from build123d import *

# Parameters (mm, degrees)
F0_W          = 40
F0_H          = 70
F1_DEPTH      = 20
F1_DEPTH_BACK = 20
F3_D          = 19.5
F5_D          = 30
F6_R          = 19.99999


# Not quite as in the source:
# - a fillet or chamfer is up to 0.001 mm smaller than in the source, because OpenCascade refuses the exact size


with BuildPart() as f1:
    # F0 (on Front) → F1 (new body, two sides)
    with BuildSketch(Plane.XZ) as f1_sk:
        Rectangle(F0_W, F0_H)
    extrude(amount=F1_DEPTH)
    extrude(f1_sk.sketch, amount=-F1_DEPTH_BACK)

    # F3 (through all)
    with Locations(Plane(origin=(-20, 0, 0), x_dir=(0, -1, 0), z_dir=(-1, 0, 0))):
        with Locations((0, 20)):
            Hole(F3_D / 2)

    # F5 (through all)
    with Locations(Plane.XZ.offset(20)):
        with Locations((0, -15)):
            Hole(F5_D / 2)

    # F6 (radius 20 in the source; OpenCascade refuses exactly that, so slightly less here)
    f6_edges = [f1.edges().sort_by_distance(p)[0] for p in [
        (20, 0, -35),
        (-20, 0, -35),
    ]]
    fillet(f6_edges, radius=F6_R)


solid = f1.part
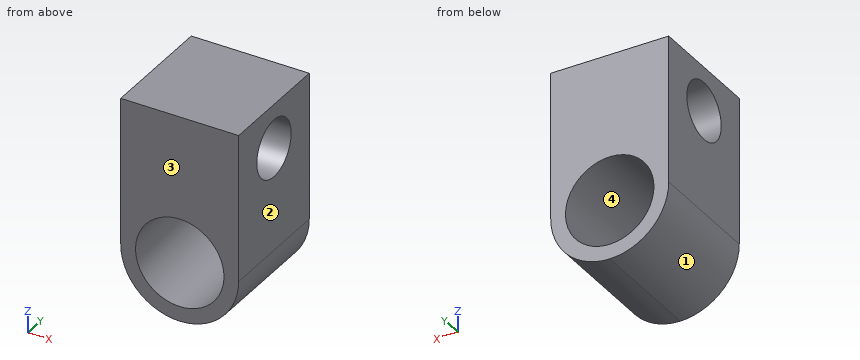
Design review of the part built by this model. Coordinates are the model's own, in mm. Face numbers are marked on the shaded views. Coordinates: 2 decimals unless noted, no trailing zeros. Order: outer loops, then holes, each group sorted by start corner. A loop starts at its lowest first (then second) coordinate and runs counter-clockwise, first axis right, second up. Notation, with made-up numbers: (-38.5, -16) - (8.5, -16) arc R32 ccw to (8.5, 10) - close; hole circle Ø8 at (-20, 2.25). An arc over 180 degrees is marked (long way). Put each result on its own line as item: value.
1) Take a section at C-C, the plane y = 0. Count the separate pieces of the cut face and the enclosed holes in it, and give its area (3 significant figures).
Response values:
separate pieces: 2
enclosed holes: 1
area: 1,140 mm²
2) The part is to be moulded in two halves that separate along X. For the marked faces 1, 2, 3 and 4, say which applies: released by +X, released by -X, zero draft, split by the parting line, or undercut.
Response values:
face 1: released by -X
face 2: released by +X
face 3: zero draft
face 4: undercut
3) Insertion check: P1, Ø1, axis at y = 10.5, z = -27, coming from the +X side; P2, Ø3, axis at y = 13, z = -21, coming from the -X side; P3, Ø18, axis at x = 0, z = -15, coming from the -Y side. Each pin has a flat end and moves straight along its axis. Give the tip position at first contact, or say it passes through.
Response values:
P1: stops at x = 16.36
P2: stops at x = -19.49
P3: passes through
4) Take a section at A-A, the plane z = 20. Give the boundary of the cut face in (x, y).
Response values:
outline: (-20, -20) - (20, -20) - (20, -9.75) - (-20, -9.75) - close; (-20, 9.75) - (20, 9.75) - (20, 20) - (-20, 20) - close
5) Take a section at B-B, the plane x = -1. Give the boundary of the cut face in (y, z).
Response values:
outline: (-20, -34.97) - (20, -34.97) - (20, -29.97) - (-20, -29.97) - close; (-20, -0.03) - (20, -0.03) - (20, 35) - (-20, 35) - close; hole circle Ø19.5 at (0, 20)
6) Wall thickness on L1, parallel to Z at x = 0, y = -3; L2, parallel to Z at x = -9, y = -8; L3, parallel to X at y = -17, z = -24.5: over which ranges is each line inside the solid? List them lowest first. Write a range as from..to.
Response values:
L1: z = -35..-30, 0..10.72, 29.28..35
L2: z = -32.86..-27, -3..14.43, 25.57..35
L3: x = -17.6..-11.61, 11.61..17.6
